```python
from build123d import *

# Parameters (mm, degrees)
SKETCH1_W                 = 3.7
SKETCH1_H                 = 12
SKETCH1_W_2               = 8
BOSS_EXTRUDE1_DEPTH       = 5
F_6_0MM_DOWEL_HOLE1_D     = 6
F_6_0MM_DOWEL_HOLE1_DEPTH = 10
F_6_0MM_DOWEL_HOLE1_TIP   = 1.802581857
CUT_EXTRUDE1_START        = -12
SKETCH5_W                 = 3.5
SKETCH5_H                 = 3.5
CUT_EXTRUDE1_DEPTH        = 12


with BuildPart() as part:
    # Sketch1 → Revolve1 (revolve)
    with BuildSketch(Plane.XY, mode=Mode.PRIVATE) as revolve1_sk:
        with Locations((6.15, 6)):
            Rectangle(SKETCH1_W, SKETCH1_H)
        with Locations((4, 18)):
            Rectangle(SKETCH1_W_2, SKETCH1_H)
    revolve(revolve1_sk.sketch.rotate(Axis((0, 0, 0), (0, 1, 0)), 90), axis=Axis((0, 0, 0), (0, 1, 0)))

    # Sketch2 → Boss-Extrude1 (add)
    with BuildSketch(Plane(origin=(0, 24, 0), x_dir=(1, 0, 0), z_dir=(0, 1, 0))):
        Polygon((6.92820323, 0), (3.464101615, 6), (-3.464101615, 6), (-6.92820323, 0), (-3.464101615, -6), (3.464101615, -6), align=None)
    extrude(amount=BOSS_EXTRUDE1_DEPTH)

    # Ø6.0mm Dowel Hole1
    with Locations(Plane(origin=(0, 29, 0), x_dir=(1, 0, 0), z_dir=(0, 1, 0))):
        with Locations((0, 0)):
            Hole(F_6_0MM_DOWEL_HOLE1_D / 2, depth=F_6_0MM_DOWEL_HOLE1_DEPTH)
            with Locations((0, 0, -(F_6_0MM_DOWEL_HOLE1_DEPTH + F_6_0MM_DOWEL_HOLE1_TIP / 2))):  # 118° drill point
                Cone(0, F_6_0MM_DOWEL_HOLE1_D / 2, F_6_0MM_DOWEL_HOLE1_TIP, mode=Mode.SUBTRACT)

    # Sketch5 → Cut-Extrude1 (cut)
    with BuildSketch(Plane.XZ.offset(CUT_EXTRUDE1_START)):
        with Locations((4.3, 0)):
            Rectangle(SKETCH5_W, SKETCH5_H)
    extrude(amount=CUT_EXTRUDE1_DEPTH, mode=Mode.SUBTRACT)


solid = part.part
```
Work out the finished part from the listing and answer in its coordinate system (mm). A direction names the side the tool comes from. Give positions to 0.01 mm unless a question says otherwise; leave off trailing zeros. Loops run counter-clockwise (first coordinate to the right, second up) from the corner with the lowest first, then second, coordinate; pieces in that order, holes last. Notation, with made-up numbers: (-8, 22) -> (35, 22) arc R10 cw to (35, 32) -> close; hole circle Ø7 at (59.5, -23.75). An arc over 180 degrees is marked (long way). Write item = value, one per line. Start each with the question number.
(1) Find section A-A on y = 2.5. Give the vertices of the cut face in (x, z).
(2) Given pin 1 Ø2.5 at (x, y) = (5, 7.5) entering from +Z; pin 2 Ø4.5 at (x, z) = (1, -1.5) entering from -Y; pin 3 Ø0.6 at (x, y) = (5, 3.5) entering from -Z, each flat-ended and moving along its own axis, determine where each tip first touches the part or whether it passes through.
(3) Find section C-C on y = 15.25. Give the vertices of the cut face in (x, z).
(4) Find section B-B on y = 22. Give the vertices of the cut face in (x, z).
(5) Which of the six approach directions +Z, -Z, +X, -X, +Y, -Y give full straight-line access (tool end or side, diameter ignored) to faces 1 (the cylindrical face through (3, 24, 0)), 2 (the flat face through (5, 6, -1.75)), 3 (the flat face through (5.22, 26.46, -2.96))?
(6) Find section D-D on y = 18.25. Give the vertices of the cut face in (x, z), and give its area (3 significant figures).
(7) The mould has two halves that part along Z. Classify faces 4 (the flat face through (1, 29, -3)), 5 (the flat face through (-5.172, 26.465, -3.042)), 6 (the flat face through (6.05, 6, 0)), 7 (the flat face through (5, 6, 1.75)): +Z half, -Z half, draft (parallel to the pull), parting line (faces both ways), or undercut.
(8) Find the intervals of material crossed by probe 1 along X at (y, z) = (4, 0); probe 2 along Z at (x, y) = (0, 26.75); probe 3 along Y at (x, z) = (-0.5, 7), in increasing order. Write a range as from..to.
From the geometry:
q1.outline = circle Ø16 at (0, 0); hole (3.93, -1.75) -> (6.05, -1.75) -> (6.05, 1.75) -> (3.93, 1.75) arc R4.3 ccw (long way) to start
q2.pin_1 = 7.07
q2.pin_2 = 12
q2.pin_3 = -6.47
q3.outline = circle Ø16 at (0, 0)
q4.outline = circle Ø16 at (0, 0); hole circle Ø6 at (0, 0)
q5.face_1 = +Y
q5.face_2 = -Y
q5.face_3 = -Z, +X, +Y
q6.outline = circle Ø16 at (0, 0); hole circle Ø3.5 at (0, 0)
q6.area = 191 mm^2
q7.face_4 = draft
q7.face_5 = -Z half
q7.face_6 = undercut
q7.face_7 = undercut
q8.probe_1 = -8..-4.3, 6.05..8
q8.probe_2 = -6..-3, 3..6
q8.probe_3 = 0..24
